Geometry check sheet. Reference: the model listing, model coordinates, mm. Face numbers are marked on the shaded views. A direction names the side the tool comes from. Round coordinates to 2 decimals unless told otherwise and drop trailing zeros. Loops run counter-clockwise (first coordinate to the right, second up) from the corner with the lowest first, then second, coordinate; pieces in that order, holes last. Notation, with made-up numbers: M 56,52.25 L 92,52.25 A25 cw 92,87.25 Z; hole C 8,-29 d4. An arc over 180 degrees is marked long. Write item = value, one per line.
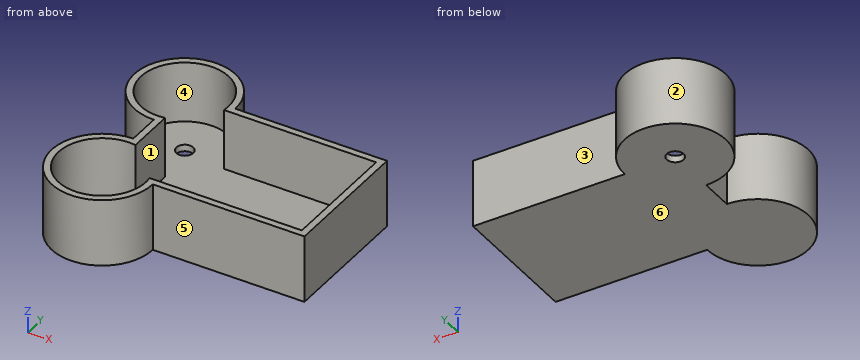
from build123d import *

# Parameters (mm, degrees)
F1_DEPTH = 25.4
F2_T     = -2.54
F4_D     = 6.35


with BuildPart() as f1:
    # F0 (on Top) → F1 (new body)
    with BuildSketch(Plane.XY):
        with BuildLine():
            Line((42.0402561671, 28.8117545512), (-15.1097438329, 28.8117545512))
            ThreePointArc((-15.1097438329, 28.8117545512), (-20.6893596513, 15.3413703696), (-34.1597438329, 9.7617545512))
            Line((-34.1597438329, 9.7617545512), (-34.1597438329, -2.9382454488))
            ThreePointArc((-34.1597438329, -2.9382454488), (-20.6893596513, -8.5178612672), (-15.1097438329, -21.9882454488))
            Line((-15.1097438329, -21.9882454488), (42.0402561671, -21.9882454488))
            Line((42.0402561671, -21.9882454488), (42.0402561671, 28.8117545512))
        make_face()
        with BuildLine():
            ThreePointArc((-15.1097438329, -21.9882454488), (-20.6893596513, -8.5178612672), (-34.1597438329, -2.9382454488))
            Line((-34.1597438329, -2.9382454488), (-34.1597438329, -21.9882454488))
            Line((-34.1597438329, -21.9882454488), (-15.1097438329, -21.9882454488))
        make_face()
        with BuildLine():
            Line((-34.1597438329, -21.9882454488), (-34.1597438329, -2.9382454488))
            ThreePointArc((-34.1597438329, -2.9382454488), (-47.6301280145, -35.4586296304), (-15.1097438329, -21.9882454488))
            Line((-15.1097438329, -21.9882454488), (-34.1597438329, -21.9882454488))
        make_face()
        with BuildLine():
            Line((-34.1597438329, 9.7617545512), (-34.1597438329, 28.8117545512))
            Line((-34.1597438329, 28.8117545512), (-15.1097438329, 28.8117545512))
            ThreePointArc((-15.1097438329, 28.8117545512), (-47.6301280145, 42.2821387328), (-34.1597438329, 9.7617545512))
        make_face()
        with BuildLine():
            Line((-15.1097438329, 28.8117545512), (-34.1597438329, 28.8117545512))
            Line((-34.1597438329, 28.8117545512), (-34.1597438329, 9.7617545512))
            ThreePointArc((-34.1597438329, 9.7617545512), (-20.6893596513, 15.3413703696), (-15.1097438329, 28.8117545512))
        make_face()
    extrude(amount=F1_DEPTH)

    # F2
    f2_openings = [f1.faces().sort_by_distance(p)[0] for p in [
        (-8.559993, 3.411755, 25.4),
    ]]
    offset(amount=F2_T, openings=f2_openings, kind=Kind.INTERSECTION)

    # F4 (through all)
    with Locations(Plane.XY.offset(2.54)):
        with Locations((-34.1597438329, 28.8117545512)):
            Hole(F4_D / 2)


solid = f1.part
(1) Tool access check on the marked faces 1, 2 and 3. Record the directions out of +Z, -Z, +X, -X, +Y, -Y that give a thin tool (end or side, any length) a straight path to the whole face; none if there is none.
Result set:
face_1 = +Z
face_2 = +Z, -Z
face_3 = +Z, -Z, +X, +Y
(2) Sectioned sample at C-C on y = 0.5. Record the cut outline in (x, z), then the cut area to 3 significant figures.
Result set:
outline = M -34.16,0 L 42.04,0 L 42.04,25.4 L 39.5,25.4 L 39.5,2.54 L -31.62,2.54 L -31.62,25.4 L -34.16,25.4 Z
area = 310 mm2
(3) Release check for a two-part mould opening along Y. For the marked faces 4, 5 and 6 record: released by +Y, released by -Y, zero draft, split by the parting line, or undercut.
Result set:
face_4 = undercut
face_5 = released by -Y
face_6 = zero draft
(4) Sectioned sample at D-D on x = -40. Record the cut outline in (y, z), then the cut area to 3 significant figures.
Result set:
outline = M -40.12,0 L -3.86,0 L -3.86,25.4 L -6.55,25.4 L -6.55,2.54 L -37.43,2.54 L -37.43,25.4 L -40.12,25.4 Z; M 10.68,0 L 46.94,0 L 46.94,25.4 L 44.25,25.4 L 44.25,2.54 L 13.37,2.54 L 13.37,25.4 L 10.68,25.4 Z
area = 430 mm2
(5) Sectioned sample at B-B on x = 15.5. Record the cut outline in (y, z), then the cut area to 3 significant figures.
Result set:
outline = M -21.99,0 L 28.81,0 L 28.81,25.4 L 26.27,25.4 L 26.27,2.54 L -19.45,2.54 L -19.45,25.4 L -21.99,25.4 Z
area = 245 mm2
(6) Depth check by flat-ended pin: pin 1 Ø8 at (x, z) = (1, 12) entering from +Y; pin 2 Ø7 at (x, z) = (15, 15) entering from -Y; pin 3 Ø10 at (y, z) = (15, 16) entering from -X. Enter the tip coordinate at first touch or a pass-through.
Result set:
pin_1 = 28.81
pin_2 = -21.99
pin_3 = -51.05
(7) Material ranges on line 1 along X through (y, z) = (8, 8.25); line 2 along Z through (x, y) = (15.5, 1); line 3 along X through (y, z) = (-20, 24.25), recorded low to high. Write a range as from..to.
Result set:
line_1 = -34.16..-31.62, 39.5..42.04
line_2 = 0..2.54
line_3 = -53.11..-50.55, -17.77..42.04
(8) Sectioned sample at A-A on z = 11.25. Record the cut outline in (x, y), then the cut area to 3 significant figures.
Result set:
outline = M -34.16,-2.94 A19.05 ccw long -15.11,-21.99 L 42.04,-21.99 L 42.04,28.81 L -15.11,28.81 A19.05 ccw long -34.16,9.76 Z; hole M -31.62,-5.67 A16.51 ccw long -17.85,-19.45 L 39.5,-19.45 L 39.5,26.27 L -17.85,26.27 A16.51 ccw long -31.62,12.5 Z
area = 891 mm2
